Model file for the job. Use its own axes, mm. Face numbers are marked on the shaded views. Coordinates: 2 decimals unless noted, no trailing zeros. Order: outer loops, then holes, each group sorted by start corner. A loop starts at its lowest first (then second) coordinate and runs counter-clockwise, first axis right, second up. Notation, with made-up numbers: (-19.75, 6.5) - (38.25, 6.5) arc R18 cw to (38.25, 41.5) - close; hole circle Ø5 at (-2.5, -38.75). An arc over 180 degrees is marked (long way). Put each result on its own line as item: value. Start each with the question number.
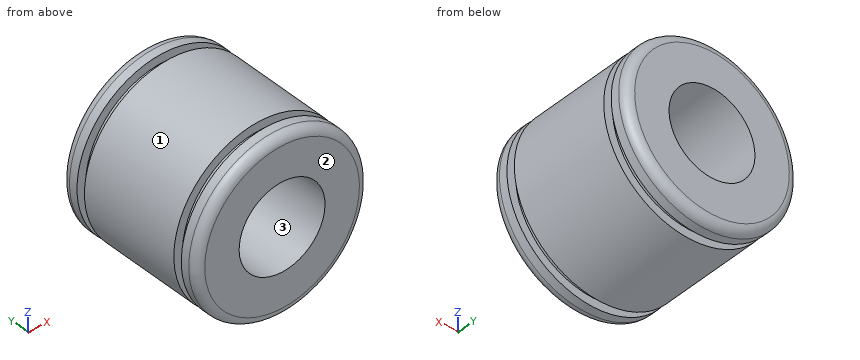
```python
from build123d import *


with BuildPart() as part:
    # Esquisse1 → Révolution1 (revolve)
    with BuildSketch(Plane.XY, mode=Mode.PRIVATE) as r_volution1_sk:
        with BuildLine():
            Line((5, 3), (5, -3))
            Line((5, -3), (4.5, -3))
            Line((4.5, -3), (4.5, -3.5))
            Line((4.5, -3.5), (5, -3.5))
            Line((5, -3.5), (5, -4))
            ThreePointArc((5, -4), (4.853553391, -4.353553391), (4.5, -4.5))
            Line((4.5, -4.5), (2.5, -4.5))
            Line((2.5, -4.5), (2.5, 4.5))
            Line((2.5, 4.5), (4.5, 4.5))
            ThreePointArc((4.5, 4.5), (4.853553391, 4.353553391), (5, 4))
            Line((5, 4), (5, 3.5))
            Line((5, 3.5), (4.5, 3.5))
            Line((4.5, 3.5), (4.5, 3))
            Line((4.5, 3), (5, 3))
        make_face()
    revolve(r_volution1_sk.sketch.rotate(Axis((0, -18.848412698, 0), (0, 1, 0)), 90), axis=Axis((0, -18.848412698, 0), (0, 1, 0)))  # turned: the seam where the file's is


solid = part.part
```
Item 1: Slice it at C-C, the plane y = -0.5. Give the cut face in (x, z), plus the area to 3 significant figures.
Item 2: Pull direction Z, two halves, no side cores. Call the marked faces 1, 2 and 3: pulls with the +Z half, pulls with the -Z half, needs draft (parallel to the pull), parting line crosses it, or undercut.
Item 3: Wall check: line 1 along X through (y, z) = (-2.5, 0); line 2 along Y through (x, z) = (-4.5, 1.25); line 3 along Z through (x, y) = (-3, -2.75). Give the ranges that are in metal, low to high.
Item 4: Flat gauge pins, fed straight in: pin 1 Ø1 at (x, y) = (-4, 2) entering from -Z; pin 2 Ø4 at (x, y) = (3, -1.5) entering from -Z; pin 3 Ø2 at (y, z) = (2, 3.5) entering from +X. Where does each tip first touch, or does it go through?
Item 5: Slice it at A-A, the plane x = 0. Give the cut face in (y, z), plus the area to 3 significant figures.
Item 6: Slice it at B-B, the plane z = 0. Give the cut face in (x, y), plus the area to 3 significant figures.
Here are the results:
1. outline: circle Ø10 at (0, 0); hole circle Ø5 at (0, 0)
1. area: 58.9 mm^2
2. face 1: parting line crosses it
2. face 2: needs draft
2. face 3: undercut
3. line 1: x = -5 to -2.5, 2.5 to 5
3. line 2: y = -4.47 to -3.5, -3 to 3, 3.5 to 4.47
3. line 3: z = -4 to 4
4. pin 1: stops at z = -3.57
4. pin 2: stops at z = -4.9
4. pin 3: stops at x = 4.33
5. outline: (-4.5, -4.5) arc R0.5 ccw to (-4, -5) - (-3.5, -5) - (-3.5, -4.5) - (-3, -4.5) - (-3, -5) - (3, -5) - (3, -4.5) - (3.5, -4.5) - (3.5, -5) - (4, -5) arc R0.5 ccw to (4.5, -4.5) - (4.5, -2.5) - (-4.5, -2.5) - close; (-4.5, 2.5) - (4.5, 2.5) - (4.5, 4.5) arc R0.5 ccw to (4, 5) - (3.5, 5) - (3.5, 4.5) - (3, 4.5) - (3, 5) - (-3, 5) - (-3, 4.5) - (-3.5, 4.5) - (-3.5, 5) - (-4, 5) arc R0.5 ccw to (-4.5, 4.5) - close
5. area: 43.8 mm^2
6. outline: (-5, -4) arc R0.5 ccw to (-4.5, -4.5) - (-2.5, -4.5) - (-2.5, 4.5) - (-4.5, 4.5) arc R0.5 ccw to (-5, 4) - (-5, 3.5) - (-4.5, 3.5) - (-4.5, 3) - (-5, 3) - (-5, -3) - (-4.5, -3) - (-4.5, -3.5) - (-5, -3.5) - close; (2.5, -4.5) - (4.5, -4.5) arc R0.5 ccw to (5, -4) - (5, -3.5) - (4.5, -3.5) - (4.5, -3) - (5, -3) - (5, 3) - (4.5, 3) - (4.5, 3.5) - (5, 3.5) - (5, 4) arc R0.5 ccw to (4.5, 4.5) - (2.5, 4.5) - close
6. area: 43.8 mm^2
